Could you check a few things on this drawing? It's one solid part, dimensions in mm from its lowest x, y, z. Give positions to 0.01 mm unless a question says otherwise; leave off trailing zeros. Loops run counter-clockwise (first coordinate to the right, second up) from the corner with the lowest first, then second, coordinate; pieces in that order, holes last. Notation, with made-up numbers: M 16,27.25 L 67,27.25 A10 ccw 67,37.25 Z; hole C 57.25,42.25 d4. An arc over 180 degrees is marked long. Answer as CSV lines item,"result". Start each with the question number.
Item 1: I want a section at B-B on z = 2.85. List the corners of the cut face in (x, y) for me, plus the area to 4 significant figures.
Item 2: I want a section at A-A on x = 40.5. List the corners of the cut face in (y, z) for me.
Item 3: I want a section at D-D on y = 29.5. List the corners of the cut face in (x, z) for me.
Item 4: If I drill on line 1 along Y through (x, z) = (28, 5); line 2 along Y through (x, z) = (46.5, 3.55); line 3 along X through (y, z) = (76.5, 3.8), over which ranges is the centre line in solid material (lowest first)? Write a range as from..to.
Item 5: I want a section at C-C on x = 13. List the corners of the cut face in (y, z) for me.
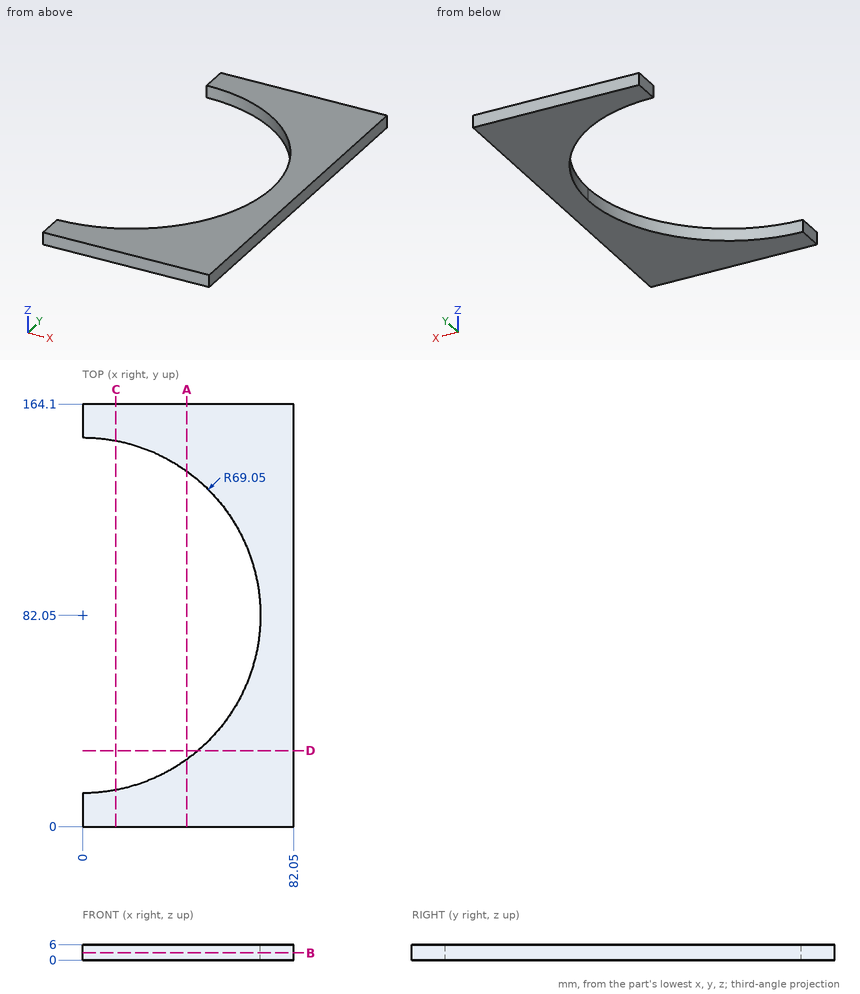
Result:
1,outline,"M 0,0 L 82.05,0 L 82.05,164.1 L 0,164.1 L 0,151.1 A69.05 cw 0,13 Z"
1,area,"5,975 mm^2"
2,outline,"M 0,0 L 26.12,0 L 26.12,6 L 0,6 Z; M 137.98,0 L 164.1,0 L 164.1,6 L 137.98,6 Z"
3,outline,"M 44.79,0 L 82.05,0 L 82.05,6 L 44.79,6 Z"
4,line 1,"0..18.93, 145.17..164.1"
4,line 2,"0..31, 133.1..164.1"
4,line 3,"68.83..82.05"
5,outline,"M 0,0 L 14.23,0 L 14.23,6 L 0,6 Z; M 149.87,0 L 164.1,0 L 164.1,6 L 149.87,6 Z"
